Solid Edge part; units mm, degrees
sketch "Sketch1" plane through (0, 0, 0) normal (0, -1, 0) x (1, 0, 0)
  line L0 (-19, 0) -> (0, 0)
  line L1 (0, 0) -> (0, -1)
  line L2 (-4, -4.5) -> (0, -1)
  line L3 (-4, -4.5) -> (-14, -6.5)
  line L4 (-14, -6.5) -> (-19, -6.5)
  line L5 (-19, 0) -> (-19, -6.5)
extrude "Protrusion1" add sketch "Sketch1" along normal mid plane 6.5
fillet "Verrundung_1" radius 2 1 edges at (-4, 0, -4.5)
hole "Bohrung_1" at (-5, 0.75, 0) direction (0, 0, -1) diameter 2.8 depth 3.6
hole "Hole1" at (-15, 0.75, 0) direction (0, 0, -1) diameter 2.8 depth 3.6
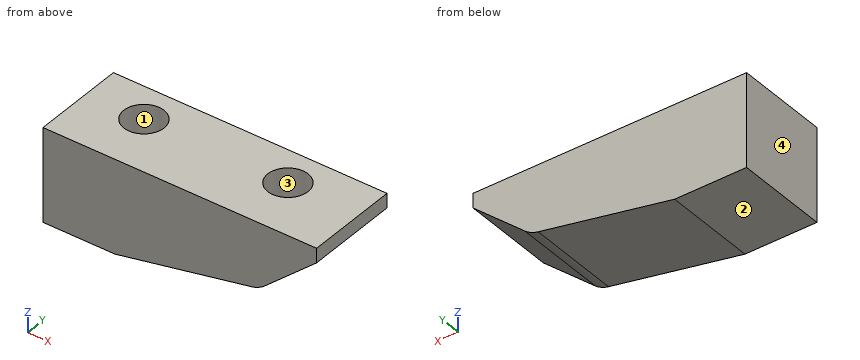
Geometry: final body of the model. Coordinates: model frame, mm. Face numbers are marked on the shaded views. Give positions to 0.01 mm unless a question says otherwise; leave off trailing zeros. Loops run counter-clockwise (first coordinate to the right, second up) from the corner with the lowest first, then second, coordinate; pieces in that order, holes last. Notation, with made-up numbers: (4.5, 15) - (26.5, 15) arc R22 cw to (26.5, 28) - close; hole circle Ø5 at (38.5, 49). An arc over 180 degrees is marked (long way). Answer as CSV lines item,"result". Start each with the question number.
(1) Section query C-C (y = 0.75). Output: boundary loops of the cut face in (x, z), and give its area (3 significant figures).
(2) Ray query, line 1 along Y through (x, z) = (-5, -1.85); line 2 along X through (y, z) = (1, -3); line 3 along X through (y, z) = (0.75, -1.8). Return the intervals inside material, ascending. Write a range as [from, to].
(3) Mould query, pull axis X, two halves, no side actions, for the marked faces 1, 2, 3 and 4. Classes: +X half, -X half, draft (parallel to the pull), parting line (faces both ways), or undercut.
(4) Section query A-A (x = -5). Output: boundary loops of the cut face in (y, z).
(5) Pin query (flat end, axial travel): P1, Ø1.7, axis at x = -15, y = 0.75, coming from the +Z side. Return the tip coordinate at first contact, or that it passes through.
(6) Section query B-B (z = -0.75). Output: boundary loops of the cut face in (x, y).
(7) Section query D-D (z = -5). Output: boundary loops of the cut face in (x, y), and give its area (4 significant figures).
Worked answers:
1,outline,"(-19, -6.5) - (-14, -6.5) - (-4.52, -4.6) arc R2 ccw to (-3.6, -4.15) - (0, -1) - (0, 0) - (-3.6, 0) - (-3.6, -3.6) - (-6.4, -3.6) - (-6.4, 0) - (-13.6, 0) - (-13.6, -3.6) - (-16.4, -3.6) - (-16.4, 0) - (-19, 0) - close"
1,area,"78.3 mm^2"
2,line 1,"y = [-3.25, -0.65], [2.15, 3.25]"
2,line 2,"x = [-19, -16.38], [-13.62, -6.38], [-3.62, -2.29]"
2,line 3,"x = [-19, -16.4], [-13.6, -6.4], [-3.6, -0.91]"
3,face 1,"undercut"
3,face 2,"draft"
3,face 3,"undercut"
3,face 4,"-X half"
4,outline,"(-3.25, -4.7) - (3.25, -4.7) - (3.25, 0) - (2.15, 0) - (2.15, -3.6) - (-0.65, -3.6) - (-0.65, 0) - (-3.25, 0) - close"
5,P1,"stops at z = -3.6"
6,outline,"(-19, -3.25) - (0, -3.25) - (0, 3.25) - (-19, 3.25) - close; hole circle Ø2.8 at (-15, 0.75); hole circle Ø2.8 at (-5, 0.75)"
7,outline,"(-19, -3.25) - (-6.5, -3.25) - (-6.5, 3.25) - (-19, 3.25) - close"
7,area,"81.25 mm^2"
